Read the model definition and answer for the solid it produces. Units are mm, in the model's axes. A direction names the side the tool comes from. Coordinates: 2 decimals unless noted, no trailing zeros. Loops run counter-clockwise (first coordinate to the right, second up) from the corner with the lowest first, then second, coordinate; pieces in that order, holes last.
Q1. Section B-B (x = 12.25) is taken. Give the vertices of the cut face in (y, z).
Q2. Section D-D (x = 19.25) is taken. Give the vertices of the cut face in (y, z), then the cut area to 3 significant figures.
Q3. Straight lines are drawn through the part: line 1 (Y direction, x = 24.55, z = 0); line 2 (Y direction, x = 18.5, z = 0.25); line 3 (X direction, y = -13.75, z = 1.5). For each, find the intervals that lie inside material, in ascending order.
Q4. Flat-ended cylindrical pins translate along their axes: P1, Ø3, axis at y = 5.5, z = -2.5, coming from the -X side; P2, Ø6, axis at x = 13, z = -1.5, coming from the -Y side; P3, Ø4.5, axis at x = 11.95, z = 0, coming from the +Y side. Find the tip coordinate at first contact, or state that the pin passes through.
Q5. Section A-A (z = 0) is taken. Give the vertices of the cut face in (x, y).
Q6. Section C-C (y = 3.5) is taken. Give the vertices of the cut face in (x, z), then the cut area to 3 significant figures.
Q7. The mould has two halves that part along Z. Classify faces 3 (the face through (8.634, 9, 0)), 4 (the face through (24, 1, 6)), 5 (the face through (10.046, 9.483, 0.601)): pulls with the +Z half, pulls with the -Z half, needs draft (parallel to the pull), parting line crosses it, or undercut.
Q8. Which of the six approach directions +Z, -Z, +X, -X, +Y, -Y give full straight-line access (tool end or side, diameter ignored) to faces 1 (the face through (23.634, -5, 0)), 2 (the face through (24.648, 6.965, 0.065))?
from build123d import *

# Parameters (mm, degrees)
BOSS_EXTRUDE1_DEPTH = 6
SKETCH2_R           = 2
CUT_EXTRUDE1_DEPTH  = 10
CUT_EXTRUDE2_REACH  = 28.579
SKETCH3_R           = 0.5


with BuildPart() as part:
    # Sketch1 → Boss-Extrude1 (new, symmetric)
    with BuildSketch(Plane.XY):
        Polygon((8.63397831, 8.469387755), (23.63397831, 8.469387755), (23.63397831, -19.530612245), (25.63397831, -19.530612245), (25.63397831, 10.469387755), (8.63397831, 10.469387755), align=None)
    extrude(amount=BOSS_EXTRUDE1_DEPTH, both=True)

    # Sketch2 → Cut-Extrude1 (cut)
    with BuildSketch(Plane(origin=(0, 10.469387755, 0), x_dir=(1, 0, 0), z_dir=(0, 1, 0))):
        with Locations(Location((11.953216886, 0, 0), (0, 0, 180))):
            Circle(SKETCH2_R)
    extrude(amount=-CUT_EXTRUDE1_DEPTH, mode=Mode.SUBTRACT)

    # Sketch3 → Cut-Extrude2 (cut, up to next)
    with BuildSketch(Plane(origin=(25.63397831, 0, 0), x_dir=(0, 0, -1), z_dir=(1, 0, 0)), mode=Mode.PRIVATE) as cut_extrude2_sk1:
        with Locations((0, -15.530612245)):
            Circle(SKETCH3_R)
    cut_extrude2_tool1 = extrude(cut_extrude2_sk1.sketch, amount=-CUT_EXTRUDE2_REACH, mode=Mode.PRIVATE) & part.part
    # Sketch3 → Cut-Extrude2 (cut, up to next)
    with BuildSketch(Plane(origin=(25.63397831, 0, 0), x_dir=(0, 0, -1), z_dir=(1, 0, 0)), mode=Mode.PRIVATE) as cut_extrude2_sk2:
        with Locations((0, 6.469387755)):
            Circle(SKETCH3_R)
    cut_extrude2_tool2 = extrude(cut_extrude2_sk2.sketch, amount=-CUT_EXTRUDE2_REACH, mode=Mode.PRIVATE) & part.part
    add(cut_extrude2_tool1.solids().sort_by_distance((25.633978, -15.530612, 0))[0], mode=Mode.SUBTRACT)
    add(cut_extrude2_tool2.solids().sort_by_distance((25.633978, 6.469388, 0))[0], mode=Mode.SUBTRACT)


solid = part.part
Numbers:
1. outline: (8.47, -6) - (10.47, -6) - (10.47, -1.98) - (8.47, -1.98) - close; (8.47, 1.98) - (10.47, 1.98) - (10.47, 6) - (8.47, 6) - close
2. outline: (8.47, -6) - (10.47, -6) - (10.47, 6) - (8.47, 6) - close
2. area: 24.0 mm2
3. line 1: y = -19.53 to -16.03, -15.03 to 5.97, 6.97 to 10.47
3. line 2: y = 8.47 to 10.47
3. line 3: x = 23.63 to 25.63
4. P1: stops at x = 23.63
4. P2: stops at y = 8.47
4. P3: stops at y = 10.47
5. outline: (8.63, 8.47) - (9.95, 8.47) - (9.95, 10.47) - (8.63, 10.47) - close; (13.95, 8.47) - (23.63, 8.47) - (23.63, 6.97) - (25.63, 6.97) - (25.63, 10.47) - (13.95, 10.47) - close; (23.63, -19.53) - (25.63, -19.53) - (25.63, -16.03) - (23.63, -16.03) - close; (23.63, -15.03) - (25.63, -15.03) - (25.63, 5.97) - (23.63, 5.97) - close
6. outline: (23.63, -6) - (25.63, -6) - (25.63, 6) - (23.63, 6) - close
6. area: 24.0 mm2
7. face 3: needs draft
7. face 4: pulls with the +Z half
7. face 5: undercut
8. face 1: +Z, -Z, -X, -Y
8. face 2: +X, -X
